Build history of the part. All positions in model axes, mm. Face numbers are marked on the shaded views. A direction names the side the tool comes from. Give positions to 0.01 mm unless a question says otherwise; leave off trailing zeros. Order: outer loops, then holes, each group sorted by start corner. A loop starts at its lowest first (then second) coordinate and runs counter-clockwise, first axis right, second up. Notation, with made-up numbers: (86.25, -21.75) -> (123.25, -21.75) arc R24 cw to (123.25, 8.25) -> close; hole circle Ø9 at (48, 76). An arc over 180 degrees is marked (long way). Write item = value, one per line. Start each with the question number.
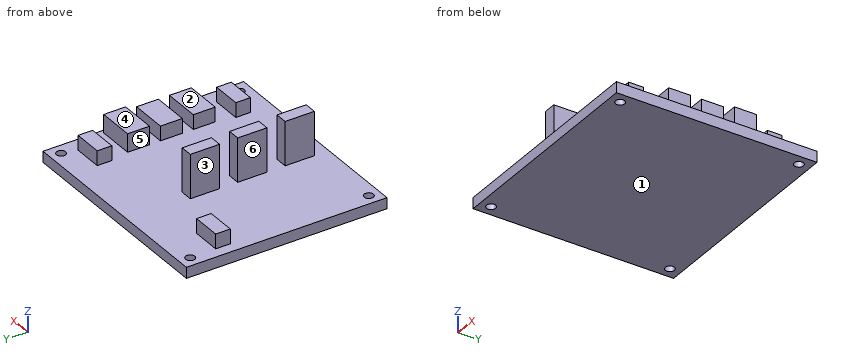
from build123d import *

# Parameters (mm, degrees)
SKETCH1_W           = 76.2
SKETCH1_H           = 69.85
BOSS_EXTRUDE1_DEPTH = 3.81
SKETCH2_R           = 1.5875
CUT_EXTRUDE1_DEPTH  = 104.440700887
SKETCH3_W           = 12.7
SKETCH3_H           = 7.62
BOSS_EXTRUDE2_DEPTH = 6.35
SKETCH3_4_W         = 10.16
SKETCH3_4_H         = 5.08
SKETCH3_4_W_2       = 12.7
SKETCH3_4_H_2       = 7.62
BOSS_EXTRUDE3_DEPTH = 5.08
SKETCH6_W           = 4.318
SKETCH6_H           = 10.16
BOSS_EXTRUDE4_DEPTH = 15.24


with BuildPart() as part:
    # Sketch1 → Boss-Extrude1 (new body)
    with BuildSketch(Plane.XY):
        with Locations((38.1, 34.925)):
            Rectangle(SKETCH1_W, SKETCH1_H)
    extrude(amount=BOSS_EXTRUDE1_DEPTH)

    # Sketch2 → Cut-Extrude1 (cut, through all)
    with BuildSketch(Plane.XY.offset(3.81)):
        with Locations((3.81, 66.04)):
            Circle(SKETCH2_R)
        with Locations((72.39, 66.04)):
            Circle(SKETCH2_R)
        with Locations((72.39, 3.81)):
            Circle(SKETCH2_R)
        with Locations((3.81, 3.81)):
            Circle(SKETCH2_R)
    extrude(amount=-CUT_EXTRUDE1_DEPTH, mode=Mode.SUBTRACT)

    # Sketch3 → Boss-Extrude2 (add)
    with BuildSketch(Plane.XY.offset(3.81)):
        with Locations((68.58, 45.72)):
            Rectangle(SKETCH3_W, SKETCH3_H)
    extrude(amount=BOSS_EXTRUDE2_DEPTH)

    # Sketch3<4> → Boss-Extrude3 (add)
    with BuildSketch(Plane.XY.offset(3.81)):
        with Locations((8.89, 54.61)):
            Rectangle(SKETCH3_4_W, SKETCH3_4_H)
        with Locations((66.04, 58.42)):
            Rectangle(SKETCH3_4_W, SKETCH3_4_H)
        with Locations((68.58, 45.72)):
            Rectangle(SKETCH3_4_W_2, SKETCH3_4_H_2)
        with Locations((68.58, 34.29)):
            Rectangle(SKETCH3_4_W_2, SKETCH3_4_H_2)
        with Locations((68.58, 22.86)):
            Rectangle(SKETCH3_4_W_2, SKETCH3_4_H_2)
        with Locations((66.04, 10.16)):
            Rectangle(SKETCH3_4_W, SKETCH3_4_H)
    extrude(amount=BOSS_EXTRUDE3_DEPTH)

    # Sketch6 → Boss-Extrude4 (add)
    with BuildSketch(Plane.XY.offset(3.81)):
        with Locations((33.02, 43.18)):
            Rectangle(SKETCH6_W, SKETCH6_H)
        with Locations((33.02, 26.67)):
            Rectangle(SKETCH6_W, SKETCH6_H)
        with Locations((33.02, 10.16)):
            Rectangle(SKETCH6_W, SKETCH6_H)
    extrude(amount=BOSS_EXTRUDE4_DEPTH)


solid = part.part
(1) Cut at C-C, the plane x = 72.39. Give the cut face in (y, z).
(2) Cut at B-B, the plane z = 12. Give the cut face in (x, y).
(3) 3-axis set-ups, long thin cutter, end or side, ignore diameter. For the marked faces 1, 2, 3 and 4: which of +Z, -Z, +X, -X, +Y, -Y reach the whole face in a straight line?
(4) Wall check: line 1 (Y direction, x = 3.81, z = 2.75); line 2 (X direction, y = 66.04, z = 2.3); line 3 (Z direction, x = 16, y = 42.5). Give the ranges that are in metal, low to high. Write a range as [from, to].
(5) Cut at A-A, the plane y = 3.81. Give the cut face in (x, z), plus the area to 3 significant figures.
(6) Cut at D-D, the plane y = 25. Give the cut face in (x, z), plus the area to 3 significant figures.
(7) Flat gauge pins, fed straight in: P1, Ø1.9, axis at y = 47.5, z = 5.5, coming from the +X side; P2, Ø1.5, axis at y = 53.5, z = 6.5, coming from the -X side; P3, Ø10, axis at y = 32, z = 15, coming from the +X side; P4, Ø6, axis at y = 61, z = 14, coming from the -X side. Where does each tip first touch, or does it go through?
(8) Mould opens along Y. For the marked faces 5 and 6 say: released by +Y, released by -Y, zero draft, split by the parting line, or undercut.
Results:
q1.outline = (0, 0) -> (2.22, 0) -> (2.22, 3.81) -> (0, 3.81) -> close; (5.4, 0) -> (64.45, 0) -> (64.45, 3.81) -> (49.53, 3.81) -> (49.53, 10.16) -> (41.91, 10.16) -> (41.91, 3.81) -> (38.1, 3.81) -> (38.1, 8.89) -> (30.48, 8.89) -> (30.48, 3.81) -> (26.67, 3.81) -> (26.67, 8.89) -> (19.05, 8.89) -> (19.05, 3.81) -> (5.4, 3.81) -> close; (67.63, 0) -> (69.85, 0) -> (69.85, 3.81) -> (67.63, 3.81) -> close
q2.outline = (30.86, 5.08) -> (35.18, 5.08) -> (35.18, 15.24) -> (30.86, 15.24) -> close; (30.86, 21.59) -> (35.18, 21.59) -> (35.18, 31.75) -> (30.86, 31.75) -> close; (30.86, 38.1) -> (35.18, 38.1) -> (35.18, 48.26) -> (30.86, 48.26) -> close
q3.face_1 = -Z, +X, -X, +Y, -Y
q3.face_2 = +Z, +X, -Y
q3.face_3 = +Z, -X, +Y, -Y
q3.face_4 = +Z, +X, +Y, -Y
q4.line_1 = [0, 2.22], [5.4, 64.45], [67.63, 69.85]
q4.line_2 = [0, 2.22], [5.4, 70.8], [73.98, 76.2]
q4.line_3 = [0, 3.81]
q5.outline = (0, 0) -> (2.22, 0) -> (2.22, 3.81) -> (0, 3.81) -> close; (5.4, 0) -> (70.8, 0) -> (70.8, 3.81) -> (5.4, 3.81) -> close; (73.98, 0) -> (76.2, 0) -> (76.2, 3.81) -> (73.98, 3.81) -> close
q5.area = 266 mm2
q6.outline = (0, 0) -> (76.2, 0) -> (76.2, 3.81) -> (74.93, 3.81) -> (74.93, 8.89) -> (62.23, 8.89) -> (62.23, 3.81) -> (35.18, 3.81) -> (35.18, 19.05) -> (30.86, 19.05) -> (30.86, 3.81) -> (0, 3.81) -> close
q6.area = 421 mm2
q7.P1 = 74.93
q7.P2 = 3.81
q7.P3 = 35.18
q7.P4 = through
q8.face_5 = undercut
q8.face_6 = zero draft
